Can you work these out from the model? Positions are in its coordinate system, mm. Face numbers are marked on the shaded views. A direction names the side the tool comes from. Give positions to 0.01 mm unless a question says otherwise; leave off trailing zeros. Write each loop counter-clockwise with the first axis right and the second up, starting at its lowest first coordinate (ties: lowest second). Pieces come first, ordered by that corner, then holes. Notation, with made-up numbers: (-27, 73.25) -> (-7, 73.25) arc R25 cw to (-7, 107.25) -> close; hole circle Ø10 at (13, 30.5). An arc over 180 degrees is marked (long way). One line per item, written item: value.
from build123d import *

# Parameters (mm, degrees)
SKETCH1_R           = 20
BOSS_EXTRUDE1_DEPTH = 50
SKETCH2_R           = 5
BOSS_EXTRUDE2_DEPTH = 10
SKETCH3_R           = 18
BOSS_EXTRUDE3_DEPTH = 1
SKETCH4_R           = 16
BOSS_EXTRUDE4_DEPTH = 5
BOSS_EXTRUDE4_TAPER = 45
SKETCH5_R           = 8
BOSS_EXTRUDE5_DEPTH = 37
BOSS_EXTRUDE6_DEPTH = 17
SKETCH7_R           = 6
BOSS_EXTRUDE7_DEPTH = 10
THREAD1_PITCH       = 2


with BuildPart() as part:
    # Sketch1 → Boss-Extrude1 (new body)
    with BuildSketch(Plane(origin=(0, 0, 0), x_dir=(0, 0, -1), z_dir=(1, 0, 0))):
        Circle(SKETCH1_R)
    extrude(amount=BOSS_EXTRUDE1_DEPTH)

    # Sketch2 → Boss-Extrude2 (add)
    with BuildSketch(Plane.ZY):
        with Locations(Location((0, 10, 0), (0, 0, 180))):
            Circle(SKETCH2_R)
        with Locations(Location((0, -10, 0), (0, 0, 180))):
            Circle(SKETCH2_R)
    extrude(amount=BOSS_EXTRUDE2_DEPTH)

    # Sketch3 → Boss-Extrude3 (add)
    with BuildSketch(Plane(origin=(50, 0, 0), x_dir=(0, 0, -1), z_dir=(1, 0, 0))):
        Circle(SKETCH3_R)
    extrude(amount=BOSS_EXTRUDE3_DEPTH)

    # Sketch4 → Boss-Extrude4 (add)
    with BuildSketch(Plane(origin=(51, 0, 0), x_dir=(0, 0, -1), z_dir=(1, 0, 0))):
        Circle(SKETCH4_R)
    extrude(amount=BOSS_EXTRUDE4_DEPTH, taper=BOSS_EXTRUDE4_TAPER)

    # Sketch5 → Boss-Extrude5 (add)
    with BuildSketch(Plane(origin=(56, 0, 0), x_dir=(0, 0, -1), z_dir=(1, 0, 0))):
        Circle(SKETCH5_R)
    extrude(amount=BOSS_EXTRUDE5_DEPTH)

    # Sketch6 → Boss-Extrude6 (add)
    with BuildSketch(Plane(origin=(93, 0, 0), x_dir=(0, 0, -1), z_dir=(1, 0, 0))):
        Polygon((6.92820323, 4), (0, 8), (-6.92820323, 4), (-6.92820323, -4), (0, -8), (6.92820323, -4), align=None)
    extrude(amount=BOSS_EXTRUDE6_DEPTH)

    # Sketch7 → Boss-Extrude7 (add)
    with BuildSketch(Plane(origin=(110, 0, 0), x_dir=(0, 0, -1), z_dir=(1, 0, 0))):
        Circle(SKETCH7_R)
    extrude(amount=BOSS_EXTRUDE7_DEPTH)

    # Thread1: the profile of Thread Profile1 profile screwed along a right-hand helix of 5 turns, 10 arcs to a turn; built about Z, then put on its axis
    thread1_z = Axis((0, 0, 0), (0, 0, 1))
    thread1_corners = [(6.0003, 0, -0.000173205), (6.0003, 0, 1.7501732), (4.91746825, 0, 1.124999997), (4.91746825, 0, 0.624999997)]
    with BuildLine(mode=Mode.PRIVATE) as thread1_profile:
        Line(thread1_corners[0], thread1_corners[1])
        Line(thread1_corners[1], thread1_corners[2])
        Line(thread1_corners[2], thread1_corners[3])
        Line(thread1_corners[3], thread1_corners[0])
    thread1_cap = Face(thread1_profile.wire())
    thread1_turn_angles = [0, 18, 36, 54, 72, 90, 108, 126, 144, 162, 180, 198, 216, 234, 252, 270, 288, 306, 324, 342, 360]
    thread1_turn_weights = [1, 0.9510565162951535, 1, 0.9510565162951535, 1, 0.9510565162951535, 1, 0.9510565162951535, 1, 0.9510565162951535, 1, 0.9510565162951535, 1, 0.9510565162951535, 1, 0.9510565162951535, 1, 0.9510565162951535, 1, 0.9510565162951535, 1]
    thread1_turn_rails = [Edge.make_bspline([Vector(p[0], p[1], 0).rotate(thread1_z, thread1_turn_angles[k]) / thread1_turn_weights[k] + Vector(0, 0, p[2] + THREAD1_PITCH * thread1_turn_angles[k] / 360) for k in range(21)], [0, 0, 0, 1, 1, 2, 2, 3, 3, 4, 4, 5, 5, 6, 6, 7, 7, 8, 8, 9, 9, 10, 10, 10], 2, thread1_turn_weights) for p in thread1_corners]
    thread1_turn_sides = [Face.make_surface_from_curves(thread1_turn_rails[p[0]], thread1_turn_rails[p[1]]) for p in [(0, 1), (1, 2), (2, 3), (3, 0)]]
    thread1 = Plane(origin=(110, 0, 0), x_dir=(0, 0, -1), z_dir=(1, 0, 0)) * Solid(Shell([*[p.moved(Location((0, 0, THREAD1_PITCH * i))) for i in range(5) for p in thread1_turn_sides], thread1_cap, thread1_cap.rotate(thread1_z, 1800).moved(Location((0, 0, THREAD1_PITCH * 1800 / 360)))]))
    add(thread1, mode=Mode.SUBTRACT)


solid = part.part
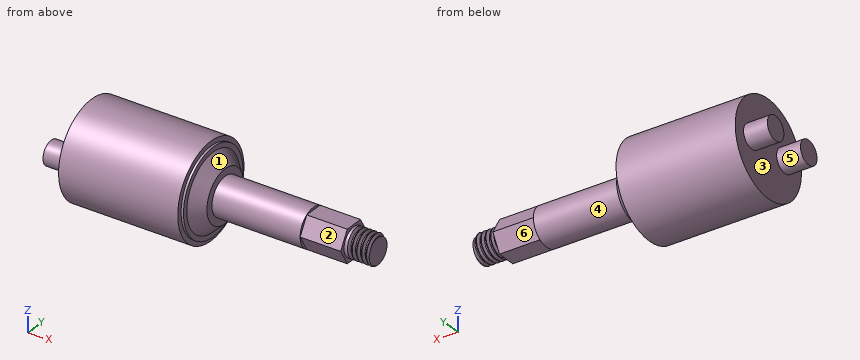
1) For the marked faces 1, 2 and 3, which set-ups out of +Z, -Z, +X, -X, +Y, -Y let a thin tool reach every point of the face, with its end or its side?
Answer list:
face 1: +X
face 2: +Z, +X, -Y
face 3: -X
2) If we section it at C-C (x = 45): Write out the boundary of the cut face in (y, z), and give its area (3 significant figures).
Answer list:
outline: circle Ø40 at (0, 0)
area: 1,260 mm^2
3) We'd pull the mould along Y, two halves only. Please class the marked faces 4, 5 and 6: released by +Y, released by -Y, zero draft, split by the parting line, or undercut.
Answer list:
face 4: split by the parting line
face 5: undercut
face 6: released by +Y
4) I need wall thicknesses on L1, parallel to X at y = -6, z = 7; L2, parallel to Y at x = 34, z = -12; L3, parallel to X at y = -7, z = 16. Which ranges of each line are inside material? Lowest first, please.
Answer list:
L1: x = 0 to 56
L2: y = -16 to 16
L3: x = 0 to 51
5) If we section it at B-B (x = 63.5): Write out the boundary of the cut face in (y, z).
Answer list:
outline: circle Ø16 at (0, 0)
6) If we section it at A-A (x = 101.5): Write out the boundary of the cut face in (y, z), and give its area (3 significant figures).
Answer list:
outline: (-8, 0) -> (-4, -6.93) -> (4, -6.93) -> (8, 0) -> (4, 6.93) -> (-4, 6.93) -> close
area: 166 mm^2
7) Will these pins go through, and if not, where does the flat tip stop? pin 1 (0.5 mm diameter, centred on y = 0, z = 7.5, fed in from +X); pin 2 (1.2 mm diameter, centred on y = 5, z = 5, fed in from +X); pin 3 (3 mm diameter, centred on y = -6, z = 3, fed in from +X); pin 4 (1.5 mm diameter, centred on x = 100.5, z = -9, fed in from +Y).
Answer list:
pin 1: stops at x = 93
pin 2: stops at x = 110
pin 3: stops at x = 119.81
pin 4: passes through
